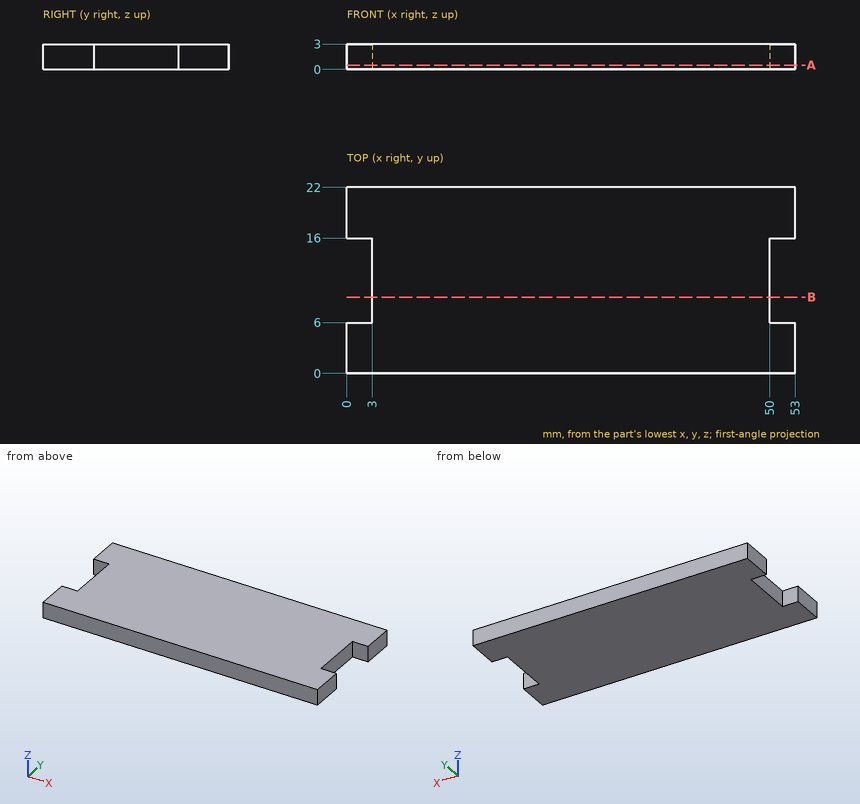
Part print with two shaded views. Sizes in mm from the minimum x, y, z corner. Give positions to 0.01 mm unless a question says otherwise; leave off trailing zeros. Order: outer loops, then holes, each group sorted by start corner. A loop starts at its lowest first (then second) coordinate and runs counter-clockwise, first axis right, second up. Notation, with made-up numbers: M -36,9 L 16,9 A27 ccw 16,40 Z; hole C -25.75,49.25 d9. An arc over 180 degrees is marked long. Put each result on its own line as item: value.
Item 1: Cut at A-A on z = 0.5. Write the cut outline in (x, y), then the cut area to 3 significant figures.
Results are:
outline: M 0,0 L 53,0 L 53,6 L 50,6 L 50,16 L 53,16 L 53,22 L 0,22 L 0,16 L 3,16 L 3,6 L 0,6 Z
area: 1,110 mm2
Item 2: Cut at B-B on y = 9. Write the cut outline in (x, z), then the cut area to 3 significant figures.
Results are:
outline: M 3,0 L 50,0 L 50,3 L 3,3 Z
area: 141 mm2
Item 3: Wall check: probe 1 along X at (y, z) = (9, 0.9). Give the ranges that are in metal, low to high.
Results are:
probe 1: 3 to 50
Item 4: Drop a flat-ended pin along its axis: pin 1 Ø0.9 at (y, z) = (12.5, 1.5) entering from +X. Give the stop position or say it passes through.
Results are:
pin 1: x = 50
